For this review, use the dimensioned drawing (mm, ordinates from the lowest corner) and the shaded views. A direction names the side the tool comes from. Round coordinates to 2 decimals unless told otherwise and drop trailing zeros. Write each loop counter-clockwise with the first axis right and the second up, starting at its lowest first coordinate (ties: lowest second). Pieces come first, ordered by that corner, then holes. Notation, with made-up numbers: (39, -22) -> (60, -22) arc R25 ccw to (60, 6) -> close; hole circle Ø5 at (26, 73). An arc over 180 degrees is marked (long way). Write each question's results on one line, items separated by ' | '. Start each with the question number.
Item 1: To check wall thickness, follow line 1 along X through (y, z) = (56, 104); line 2 along X through (y, z) = (34, 56.5). State the ranges of each line that lie inside material, in increasing order.
Item 2: Clearance check with flat-ended pins moving along their axes: pin 1 (1.2 mm diameter, centred on x = 3, y = 16, fed in from +Z); pin 2 (2 mm diameter, centred on y = 47.5, z = 76.5, fed in from -X); pin 3 (4.5 mm diameter, centred on x = 2.5, y = 39.5, fed in from -Z). State where each tip first meets the part, or that it passes through.
Item 3: Add section B-B (z = 17.5). State the section outline as (x, y) points.
Item 4: The part is to be moulded in two halves that separate along Z. For the marked faces 1, 2 and 3, say which applies: +Z half, -Z half, draft (parallel to the pull), parting line (faces both ways), or undercut.
Item 5: Add section A-A (y = 56.5). State the section outline as (x, z) points.
Item 6: Tool access review of the marked faces 4, 5 and 6: name each direction out of +Z, -Z, +X, -X, +Y, -Y from which nothing blocks a thin tool from reaching the whole face with its end or side.
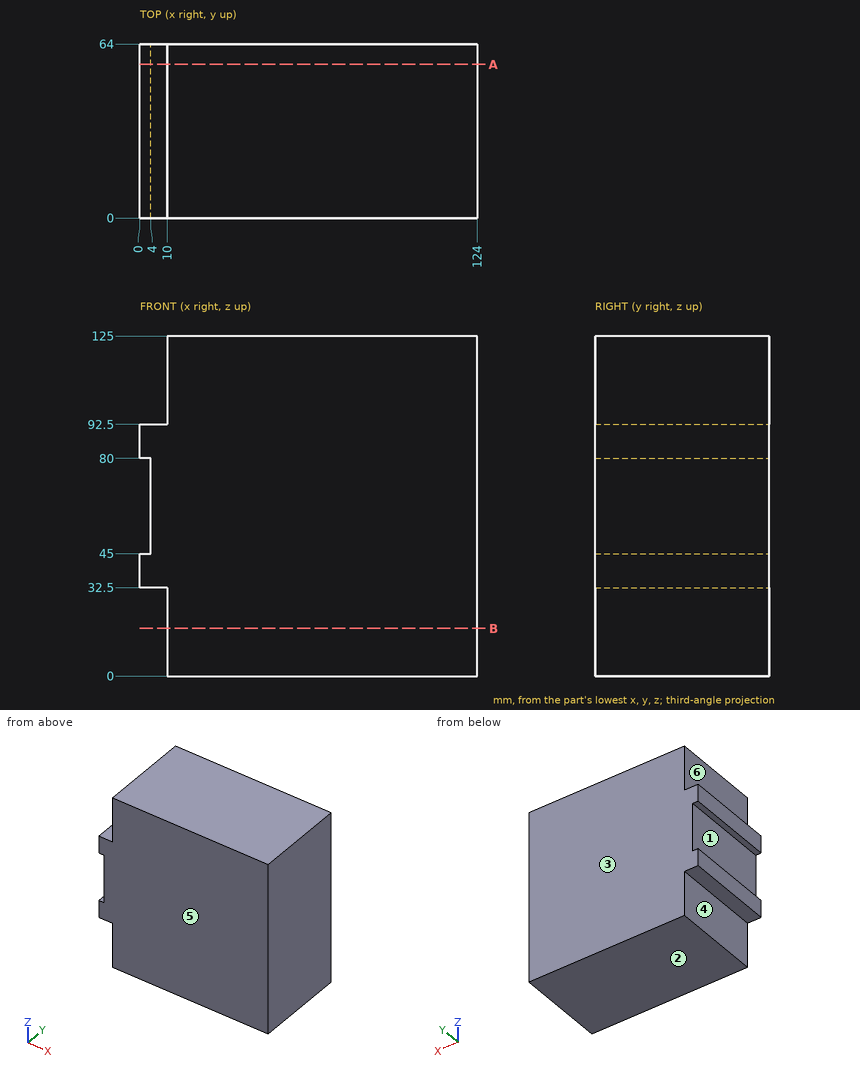
Responses:
1) line 1: x = 10 to 124 | line 2: x = 4 to 124
2) pin 1: stops at z = 92.5 | pin 2: stops at x = 4 | pin 3: stops at z = 32.5
3) outline: (10, 0) -> (124, 0) -> (124, 64) -> (10, 64) -> close
4) face 1: undercut | face 2: -Z half | face 3: draft
5) outline: (0, 32.5) -> (10, 32.5) -> (10, 0) -> (124, 0) -> (124, 125) -> (10, 125) -> (10, 92.5) -> (0, 92.5) -> (0, 80) -> (4, 80) -> (4, 45) -> (0, 45) -> close
6) face 4: -Z, -X, +Y, -Y | face 5: +Z, -Z, +X, -X, -Y | face 6: +Z, -X, +Y, -Y
